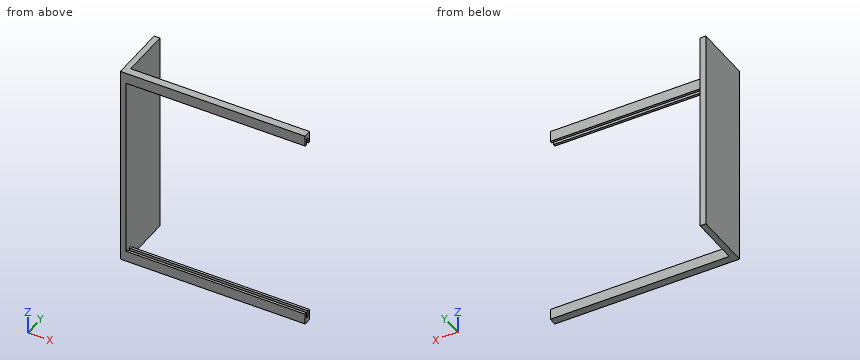
```python
from build123d import *

# Parameters (mm, degrees)
BOSS_EXTRUDE1_DEPTH = 105
CUT_EXTRUDE1_DEPTH  = 100


with BuildPart() as part:
    # Sketch1 → Boss-Extrude1 (new body)
    with BuildSketch(Plane.XY):
        Polygon((0, 26), (0, 0), (92, 0), (92, -4), (-3, -4), (-3, 26), align=None)
    extrude(amount=-BOSS_EXTRUDE1_DEPTH)

    # Sketch2 → Cut-Extrude1 (cut)
    with BuildSketch(Plane(origin=(0, 0, 0), x_dir=(0, 0, -1), z_dir=(1, 0, 0))):
        Polygon((99.5, -1.23), (102.5, -1.23), (102.5, -2.77), (99.5, -2.77), (99.5, -4), (5.5, -4), (5.5, -2.77), (2.5, -2.77), (2.5, -1.23), (5.5, -1.23), (5.5, 0), (99.5, 0), align=None)
    extrude(amount=CUT_EXTRUDE1_DEPTH, mode=Mode.SUBTRACT)


solid = part.part
```
Check sheet for the modelled part. Datum: model origin and axes. Units: mm. Coordinates: 2 decimals unless noted, no trailing zeros. Write each loop counter-clockwise with the first axis right and the second up, starting at its lowest first coordinate (ties: lowest second). Pieces come first, ordered by that corner, then holes. Notation, with made-up numbers: (-5, -8) - (13, -8) arc R18 cw to (13, 9) - close; hole circle Ø6 at (81.5, -20). An arc over 180 degrees is marked (long way). One line per question, with ' | ' between items.
Item 1: Sectioned sample at B-B on z = -7. Record the boundary of the cut face in (x, y).
Determined:
outline: (-3, -4) - (0, -4) - (0, 26) - (-3, 26) - close
Item 2: Sectioned sample at A-A on x = 64. Record the boundary of the cut face in (y, z).
Determined:
outline: (-4, -105) - (0, -105) - (0, -99.5) - (-1.23, -99.5) - (-1.23, -102.5) - (-2.77, -102.5) - (-2.77, -99.5) - (-4, -99.5) - close; (-4, -5.5) - (-2.77, -5.5) - (-2.77, -2.5) - (-1.23, -2.5) - (-1.23, -5.5) - (0, -5.5) - (0, 0) - (-4, 0) - close
Item 3: Sectioned sample at C-C on y = 20.5. Record the boundary of the cut face in (x, z).
Determined:
outline: (-3, -105) - (0, -105) - (0, 0) - (-3, 0) - close
Item 4: Gauge pin test, flat end, axial feed: P1, Ø1.6, axis at x = 61.5, z = -4, coming from the +Y side. Record the tip position at first contact, or that the pin passes through.
Determined:
P1: stops at y = 0
Item 5: Thickness scan on line 1 (Z direction, x = 44.5, y = -2.5); line 2 (Z direction, x = 80, y = -0.5); line 3 (X direction, y = 3.5, z = -21). Record the ranges inside material, lowest first. Write a range as [from, to].
Determined:
line 1: z = [-105, -102.5], [-2.5, 0] | line 2: z = [-105, -99.5], [-5.5, 0] | line 3: x = [-3, 0]
